Autodesk Fusion 360 part; units mm, degrees
sketch "Sketch1" plane through (0, 0, 0) normal (0, 0, 1) x (1, 0, 0)
  circle A0 centre (0, 0) radius 20.5
  circle A1 centre (0, 0) radius 2.5
  line L0 (2.5007, 3.5) -> (2.5007, 17.1309)
  line L1 (-2.4993, 17.135) -> (-2.4993, 3.5)
  line L2 (3.5007, 2.5) -> (17.1454, 2.5)
  line L3 (17.1398, -2.5) -> (3.5007, -2.5)
  line L4 (2.5007, 0.0585) -> (2.4993, 0.0585)
  line L5 (-2.4993, -3.5) -> (-2.4993, -17.0978)
  line L6 (2.5007, -17.1125) -> (2.5007, -3.5)
  line L7 (-3.4993, 2.5) -> (-17.1847, 2.5)
  line L8 (-17.1351, -2.5) -> (-3.4993, -2.5)
  arc A2 (-3.4993, 2.5) -> (-2.4993, 3.5) centre (-3.4993, 3.5) ccw
  arc A3 (2.5007, 3.5) -> (3.5007, 2.5) centre (3.5007, 3.5) ccw
  arc A4 (3.5007, -2.5) -> (2.5007, -3.5) centre (3.5007, -3.5) ccw
  arc A5 (-2.4993, -3.5) -> (-3.4993, -2.5) centre (-3.4993, -3.5) ccw
  line L9 (3.6805, 18.1146) -> (4.1439, 18.0299)
  arc A6 (3.6805, 18.1146) -> (2.5007, 17.1309) centre (3.5007, 17.1309) ccw
  line L10 (-3.6759, 18.1193) -> (-4.0285, 18.0561)
  arc A7 (-2.4993, 17.135) -> (-3.6759, 18.1193) centre (-3.4993, 17.135) ccw
  line L11 (-18.1755, 3.6351) -> (-18.1744, 3.6434)
  arc A8 (-18.1755, 3.6351) -> (-17.1847, 2.5) centre (-17.1847, 3.5) ccw
  line L12 (-18.1194, -3.6764) -> (-18.0575, -4.0219)
  arc A9 (-17.1351, -2.5) -> (-18.1194, -3.6764) centre (-17.1351, -3.5) ccw
  line L13 (-3.7055, -18.0763) -> (-5.1082, -17.7808)
  line L14 (3.6951, -18.0935) -> (4.6802, -17.8982)
  arc A10 (-3.7055, -18.0763) -> (-2.4993, -17.0978) centre (-3.4993, -17.0978) ccw
  arc A11 (2.5007, -17.1125) -> (3.6951, -18.0935) centre (3.5007, -17.1125) ccw
  line L15 (18.1311, 3.6681) -> (18.123, 3.7158)
  line L16 (18.1248, -3.6726) -> (18.088, -3.8826)
  arc A12 (18.1248, -3.6726) -> (17.1398, -2.5) centre (17.1398, -3.5) ccw
  arc A13 (17.1454, 2.5) -> (18.1311, 3.6681) centre (17.1454, 3.5) ccw
  arc A14 (18.123, 3.7158) -> (4.1439, 18.0299) centre (0, 0) ccw
  arc A15 (4.6802, -17.8982) -> (18.088, -3.8826) centre (0, 0) ccw
  arc A16 (-4.0285, 18.0561) -> (-18.1814, 3.4188) centre (0, 0) ccw
  arc A17 (-18.0575, -4.0219) -> (-5.1082, -17.7808) centre (0, 0) ccw
  line L17 (2.4993, 0.0585) -> (2.5007, 0.0585)
  dimension "d1" = 41
  dimension "d2" = 37
  dimension "d3" = 5
  dimension "d8" = 1
  dimension "d9" = 1
  dimension "d10" = 1
  dimension "d11" = 1
  dimension "d12" = 1
  dimension "d13" = 1
  dimension "d14" = 1
  dimension "d15" = 1
  dimension "d16" = 1
  dimension "d17" = 1
  dimension "d18" = 1
  dimension "d19" = 1
extrude "Extrude1" add sketch "Sketch1" along normal blind 3
Check sheet for the modelled part. Datum: model origin and axes. Units: mm. A direction names the side the tool comes from. Give positions to 0.01 mm unless a question says otherwise; leave off trailing zeros. Write each loop counter-clockwise with the first axis right and the second up, starting at its lowest first coordinate (ties: lowest second). Pieces come first, ordered by that corner, then holes.
Item 1: Cross-section at C-C (y = -15.5). Enter the section's corners in (x, z).
Item 2: Gauge pin test, flat ends, axial feed: pin 1 (1.5 mm diameter, centred on y = -13, z = 1.5, fed in from +X); pin 2 (1.5 mm diameter, centred on y = 9.5, z = 2, fed in from -X); pin 3 (1.5 mm diameter, centred on y = 7, z = 1.5, fed in from +X). Record the tip position at first contact, or that the pin passes through.
Item 3: Cross-section at A-A (y = 0). Enter the section's corners in (x, z).
Item 4: Access from +Z, -Z, +X, -X, +Y, -Y to the whole of each face (thin tool, end or side, straight path). Record for faces 5 (the face through (0, -4, 3)), 6 (the face through (-3, 18, 1)).
Item 5: Cross-section at D-D (z = 2). Count the separate pieces of the cut face and the enclosed holes in it, and give its area (3 significant figures).
Item 6: Draft check along X on faces 1 (the face through (13.13, 13.03, 1.48)), 2 (the face through (-17.9, 2.8, 1.5)), 3 (the face through (0, -4, 0)), 4 (the face through (-4.444, 20.013, 1.479)). Enter one of: released by +X, released by -X, zero draft, split by the parting line, or undercut.
Item 7: Scan lines: L1, parallel to Y at x = 0, z = 1.9; L2, parallel to Y at x = -3, z = 1.8; L3, parallel to Y at x = 3.5, z = 2.3. Record each from-to range of solid material in increasing order.
Report:
1. outline: (-13.42, 0) - (-10.1, 0) - (-10.1, 3) - (-13.42, 3) - close; (-2.5, 0) - (2.5, 0) - (2.5, 3) - (-2.5, 3) - close; (10.1, 0) - (13.42, 0) - (13.42, 3) - (10.1, 3) - close
2. pin 1: stops at x = 16.44
2. pin 2: stops at x = -18.54
2. pin 3: stops at x = 19.52
3. outline: (-20.5, 0) - (-2.5, 0) - (-2.5, 3) - (-20.5, 3) - close; (2.5, 0) - (20.5, 0) - (20.5, 3) - (2.5, 3) - close
4. face 5: +Z, +X, -X, +Y, -Y
4. face 6: +Z, -Z
5. separate pieces: 1
5. enclosed holes: 5
5. area: 573 mm2
6. face 1: undercut
6. face 2: undercut
6. face 3: zero draft
6. face 4: split by the parting line
7. L1: y = -20.5 to -2.5, 2.5 to 20.5
7. L2: y = -20.28 to -17.96, -2.63 to 2.63, 18 to 20.28
7. L3: y = -20.2 to -18.11, -2.5 to 2.5, 18.13 to 20.2
